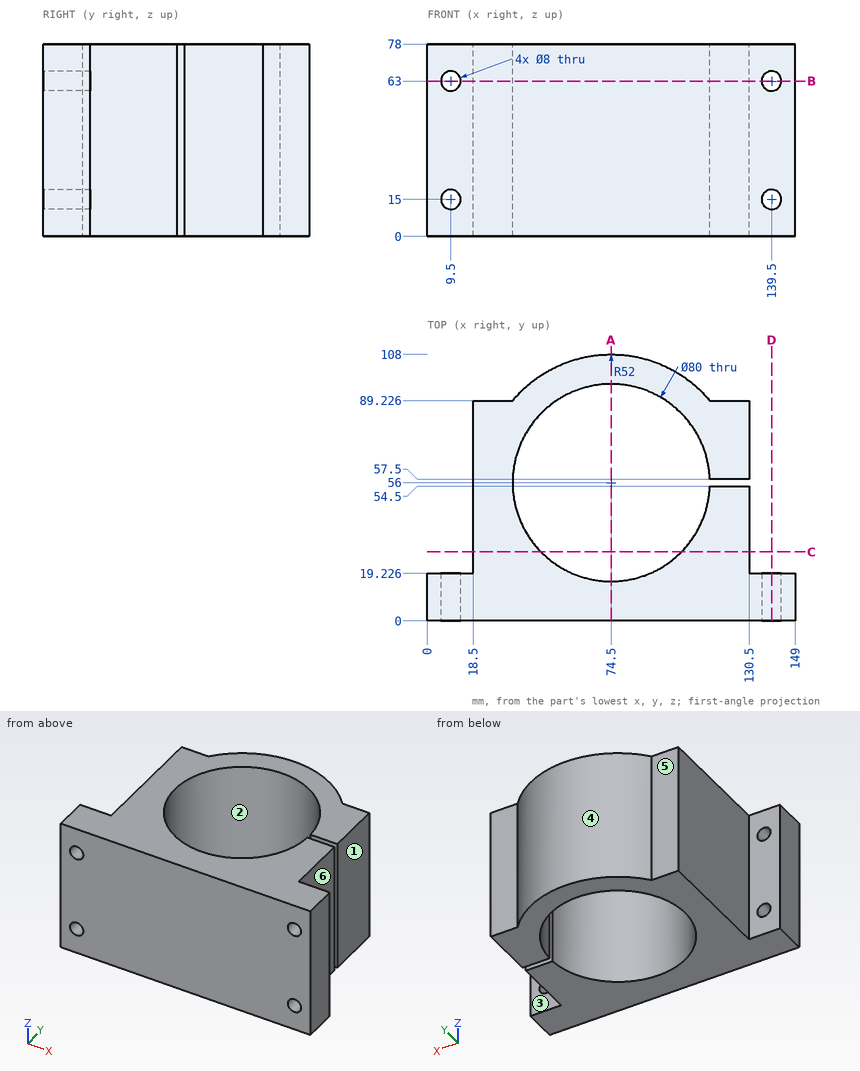
Verification items for this drawing (mm, ordinates from the low corner). A direction names the side the tool comes from. Give positions to 0.01 mm unless a question says otherwise; leave off trailing zeros. Loops run counter-clockwise (first coordinate to the right, second up) from the corner with the lowest first, then second, coordinate; pieces in that order, holes last. Notation, with made-up numbers: M 10.25,4.5 L 45.25,4.5 A26 ccw 45.25,37.5 Z; hole C -10,6.25 d3. An arc over 180 degrees is marked long. Answer as a JSON object with one key per item and string values. Group by question number.
Q1. Go/stop test with flat-tipped pins: P1, Ø13, axis at x = 29.5, z = 45.5, coming from the +Y side (1 decimal); P2, Ø3, axis at y = 59, z = 20.5, coming from the +X side; P3, Ø12, axis at x = 52.5, z = 46, coming from the -Y side; P4, Ø1, axis at x = 80.5, z = 22.5, coming from the +Y side. Record where each tip stops, or that it passes through.
Q2. Access from +Z, -Z, +X, -X, +Y, -Y to the whole of each face (thin tool, end or side, straight path). Record for the marked faces 4, 5 and 6.
Q3. Material ranges on line 1 along Z through (x, y) = (9.5, 13.25); line 2 along Z through (x, y) = (141, 17.5); line 3 along X through (y, z) = (24, 66), recorded low to high. Write a range as [from, to].
Q4. Cross-section at A-A on x = 74.5. Record the cut outline in (y, z).
Q5. Cross-section at D-D on x = 139.5. Record the cut outline in (y, z).
Q6. Release check for a two-part mould opening along Y. For the marked faces 1, 2 and 3 record: released by +Y, released by -Y, zero draft, split by the parting line, or undercut.
Q7. Cross-section at C-C on y = 28. Record the cut outline in (x, z) (1 decimal), then the cut area to 3 significant figures.
Q8. Cross-section at B-B on z = 63. Record the cut outline in (x, y), then the cut area to 3 significant figures.
Evaluation:
{
 "1": {"P1": "stops at y = 91", "P2": "stops at x = 130.5", "P3": "stops at y = 0", "P4": "stops at y = 107.71"},
 "2": {"face 4": "+Z, -Z, +Y", "face 5": "+Z, -Z, -X, +Y", "face 6": "+Z, -Z, +X, +Y"},
 "3": {"line 1": "z = [0, 11], [19, 59], [67, 78]", "line 2": "z = [0, 11.29], [18.71, 59.29], [66.71, 78]", "line 3": "x = [18.5, 50.5], [98.5, 130.5]"},
 "4": {"outline": "M 0,0 L 16,0 L 16,78 L 0,78 Z; M 96,0 L 108,0 L 108,78 L 96,78 Z"},
 "5": {"outline": "M 0,0 L 19.23,0 L 19.23,11 L 0,11 Z; M 0,19 L 19.23,19 L 19.23,59 L 0,59 Z; M 0,67 L 19.23,67 L 19.23,78 L 0,78 Z"},
 "6": {"face 1": "zero draft", "face 2": "undercut", "face 3": "released by +Y"},
 "7": {"outline": "M 18.5,0 L 45.9,0 L 45.9,78 L 18.5,78 Z; M 103.1,0 L 130.5,0 L 130.5,78 L 103.1,78 Z", "area": "4,280 mm2"},
 "8": {"outline": "M 0,0 L 5.5,0 L 5.5,19.23 L 0,19.23 Z; M 13.5,0 L 135.5,0 L 135.5,19.23 L 130.5,19.23 L 130.5,54.5 L 114.47,54.5 A40 cw long 114.47,57.5 L 130.5,57.5 L 130.5,89.23 L 114.5,89.23 A52 ccw 34.5,89.23 L 18.5,89.23 L 18.5,19.23 L 13.5,19.23 Z; M 143.5,0 L 149,0 L 149,19.23 L 143.5,19.23 Z", "area": "6,370 mm2"}
}
